```python
from build123d import *

# Parameters (mm, degrees)
SKETCH_1_W          = 18.5
SKETCH_1_H          = 8.25
EXTRUDE_1_DEPTH     = 15
SKETCH_2_R          = 3.75
EXTRUDE_2_DEPTH     = 2
SKETCH_3_R          = 2.25
EXTRUDE_3_DEPTH     = 2
SKETCH_4_R          = 1.9
EXTRUDE_4_DEPTH     = 3.3
SKETCH_5_W          = 2
SKETCH_5_H          = 0.6
EXTRUDE_5_DEPTH     = 1
SKETCH_6_W          = 25.5
SKETCH_6_H          = 8.25
EXTRUDE_6_DEPTH     = 1
SKETCH_7_R          = 1
CUT_EXTRUDE_1_DEPTH = 12.15
FILLET_1_R          = 2
SKETCH_8_W          = 5.807515018
SKETCH_8_H          = 9.098766066
CUT_EXTRUDE_2_DEPTH = 2


with BuildPart() as part:
    # 草图1 → 凸台-拉伸1 (new body)
    with BuildSketch(Plane(origin=(0, 0, 0), x_dir=(1, 0, 0), z_dir=(0, 1, 0))):
        Rectangle(SKETCH_1_W, SKETCH_1_H)
    extrude(amount=EXTRUDE_1_DEPTH)

    # 草图2 → 凸台-拉伸2 (add)
    with BuildSketch(Plane(origin=(0, 15, 0), x_dir=(1, 0, 0), z_dir=(0, 1, 0))):
        with Locations((5.5, 0)):
            Circle(SKETCH_2_R)
    extrude(amount=EXTRUDE_2_DEPTH)

    # 草图3 → 凸台-拉伸3 (add)
    with BuildSketch(Plane(origin=(0, 15, 0), x_dir=(1, 0, 0), z_dir=(0, 1, 0))):
        with Locations((1.5, 0)):
            Circle(SKETCH_3_R)
    extrude(amount=EXTRUDE_3_DEPTH)

    # 草图4 → 凸台-拉伸4 (add)
    with BuildSketch(Plane(origin=(0, 17, 0), x_dir=(1, 0, 0), z_dir=(0, 1, 0))):
        with Locations((5.5, 0)):
            Circle(SKETCH_4_R)
    extrude(amount=EXTRUDE_4_DEPTH)

    # 草图5 → 凸台-拉伸5 (add)
    with BuildSketch(Plane(origin=(9.25, 0, 0), x_dir=(0, 0, -1), z_dir=(1, 0, 0))):
        with Locations((0, 3.8)):
            Rectangle(SKETCH_5_W, SKETCH_5_H)
    extrude(amount=EXTRUDE_5_DEPTH)

    # 草图6 → 凸台-拉伸6 (add)
    with BuildSketch(Plane(origin=(0, 10.15, 0), x_dir=(1, 0, 0), z_dir=(0, 1, 0))):
        Rectangle(SKETCH_6_W, SKETCH_6_H)
    extrude(amount=EXTRUDE_6_DEPTH)

    # 草图7 → 切除-拉伸1 (cut, through all)
    with BuildSketch(Plane(origin=(0, 11.15, 0), x_dir=(1, 0, 0), z_dir=(0, 1, 0))):
        with Locations((-10.95, 0)):
            Circle(SKETCH_7_R)
        with Locations((10.95, 0)):
            Circle(SKETCH_7_R)
    extrude(amount=-CUT_EXTRUDE_1_DEPTH, mode=Mode.SUBTRACT)

    # 圆角1
    fillet_1_edges = [part.edges().sort_by_distance(p)[0] for p in [
        (-12.75, 10.65, 4.125),
        (12.75, 10.65, -4.125),
        (-12.75, 10.65, -4.125),
        (12.75, 10.65, 4.125),
    ]]
    fillet(fillet_1_edges, radius=FILLET_1_R)

    # 草图8 → 切除-拉伸2 (cut)
    with BuildSketch(Plane(origin=(0, 11.15, 0), x_dir=(1, 0, 0), z_dir=(0, 1, 0))):
        with Locations((-12.153757509, 0.424383033)):
            Rectangle(SKETCH_8_W, SKETCH_8_H)
    extrude(amount=-CUT_EXTRUDE_2_DEPTH, mode=Mode.SUBTRACT)


solid = part.part
```
The model under review builds one solid part; all positions refer to its coordinate system, in mm. A direction names the side the tool comes from. Round coordinates to 2 decimals unless told otherwise and drop trailing zeros. Loops run counter-clockwise (first coordinate to the right, second up) from the corner with the lowest first, then second, coordinate; pieces in that order, holes last. Notation, with made-up numbers: (58.5, 42.25) -> (95.5, 42.25) arc R27 ccw to (95.5, 66.25) -> close; hole circle Ø8 at (0.5, 16). An arc over 180 degrees is marked (long way). Answer as a JSON object with one key per item and string values. Group by question number.
1) For line 1 (X direction, y = 10.95, z = 0); line 2 (X direction, y = 8.25, z = 2); line 3 (Y direction, x = 3.25, z = -0.25), list the stretches that pass through material, from the lowest coordinate up. Write a range as [from, to].
2) We need section A-A on x = 7.75. Write out the cut boundary in (y, z) (3 decimals).
3) We need section D-D on x = 1.5. Write out the cut boundary in (y, z) (3 decimals), then the cut area to 3 significant figures.
4) For faces 4 (the face through (9.248, 15.986, 0.134)), 5 (the face through (1, 7, 4.125)), 6 (the face through (-9.25, 7, 0)), 7 (the face through (9.8, 11.15, -0.1)), 8 (the face through (9.6, 4.1, 0)), list the 3-axis set-ups (+Z, -Z, +X, -X, +Y, -Y) from which the entire face can be reached by the end or side of a thin tool; tool diameter is ignored.
5) We need section C-C on z = 3.25. Write out the cut boundary in (x, y).
6) We need section B-B on y = 12.5. Write out the cut boundary in (x, z) (3 decimals), then the cut area to 3 significant figures.
7) Mouldability with a two-part tool opening along Y and no side actions: class faces 1 (the face through (-2, 15, 0)), 2 (the face through (1, 7, -4.125)), 3 (the face through (9.25, 5, 0)) as released by +Y, released by -Y, zero draft, split by the parting line, or undercut.
8) For pin 1 Ø2.5 at (x, z) = (-0.5, -1) entering from +Y; pin 2 Ø3 at (x, z) = (11.5, 2) entering from -Y; pin 3 Ø2 at (y, z) = (3.5, -1.5) entering from +X, all flat-tipped, find the tip position at first contact; note any pin that passes through.
Result set:
{
 "1": {"line 1": "[-9.25, 9.95], [11.95, 12.75]", "line 2": "[-9.25, 9.25]", "line 3": "[0, 17]"},
 "2": {"outline": "(0, -4.125) -> (15, -4.125) -> (15, -3) -> (17, -3) -> (17, 3) -> (15, 3) -> (15, 4.125) -> (0, 4.125) -> close"},
 "3": {"outline": "(0, -4.125) -> (15, -4.125) -> (15, -2.25) -> (17, -2.25) -> (17, 2.25) -> (15, 2.25) -> (15, 4.125) -> (0, 4.125) -> close", "area": "133 mm²"},
 "4": {"face 4": "+Y", "face 5": "+Z, +X, -X, +Y, -Y", "face 6": "+Z, -Z, -X, +Y, -Y", "face 7": "+Z, -Z, +X, +Y", "face 8": "+Z, -Z, +X"},
 "5": {"outline": "(-9.25, 0) -> (9.25, 0) -> (9.25, 10.15) -> (12.4, 10.15) -> (12.4, 11.15) -> (9.25, 11.15) -> (9.25, 15) -> (7.37, 15) -> (7.37, 17) -> (3.63, 17) -> (3.63, 15) -> (-9.25, 15) -> close"},
 "6": {"outline": "(-9.25, -4.125) -> (9.25, -4.125) -> (9.25, 4.125) -> (-9.25, 4.125) -> close", "area": "153 mm²"},
 "7": {"face 1": "released by +Y", "face 2": "zero draft", "face 3": "undercut"},
 "8": {"pin 1": "y = 17", "pin 2": "y = 10.15", "pin 3": "x = 10.25"}
}
